from build123d import *

# Parameters (mm, degrees)
CROQUIS1_W              = 56
CROQUIS1_H              = 56
CROQUIS1_R              = 4
CROQUIS1_R_2            = 1.6
SALIENTE_EXTRUIR1_DEPTH = 5
CROQUIS2_W              = 56
CROQUIS2_H              = 3
SALIENTE_EXTRUIR2_DEPTH = 20
CROQUIS3_R              = 4.2
CORTAR_EXTRUIR1_DEPTH   = 68.416615163
CROQUIS4_R              = 2.75
CORTAR_EXTRUIR2_DEPTH   = 3
CROQUIS7_W              = 8
CROQUIS7_H              = 10
SALIENTE_EXTRUIR3_DEPTH = 5
CROQUIS5_R              = 5
CORTAR_EXTRUIR3_DEPTH   = 47.829477896
CHAFL_N1_SIZE           = 2
CHAFL_N2_SIZE           = 1.5


with BuildPart() as part:
    # Croquis1 → Saliente-Extruir1 (new body)
    with BuildSketch(Plane.XY):
        Rectangle(CROQUIS1_W, CROQUIS1_H)
        Circle(CROQUIS1_R, mode=Mode.SUBTRACT)
        with Locations((0, 11)):
            Circle(CROQUIS1_R_2, mode=Mode.SUBTRACT)
        with Locations((11, 0)):
            Circle(CROQUIS1_R_2, mode=Mode.SUBTRACT)
        with Locations((0, -11)):
            Circle(CROQUIS1_R_2, mode=Mode.SUBTRACT)
        with Locations((-11, 0)):
            Circle(CROQUIS1_R_2, mode=Mode.SUBTRACT)
    extrude(amount=SALIENTE_EXTRUIR1_DEPTH)

    # Croquis2 → Saliente-Extruir2 (add)
    with BuildSketch(Plane.XY.offset(5)):
        with Locations((0, 26.5)):
            Rectangle(CROQUIS2_W, CROQUIS2_H)
        with Locations((0, -26.5)):
            Rectangle(CROQUIS2_W, CROQUIS2_H)
    extrude(amount=SALIENTE_EXTRUIR2_DEPTH)

    # Croquis3 → Cortar-Extruir1 (cut, through all)
    with BuildSketch(Plane(origin=(0, 28, 0), x_dir=(1, 0, 0), z_dir=(0, 1, 0))):
        with Locations(Location((0, -15, 0), (0, 0, 270))):
            Circle(CROQUIS3_R)
    extrude(amount=-CORTAR_EXTRUIR1_DEPTH, mode=Mode.SUBTRACT)

    # Croquis4 → Cortar-Extruir2 (cut)
    with BuildSketch(Plane.XY.offset(5)):
        with Locations((-11, 0)):
            Circle(CROQUIS4_R)
        with Locations((0, 11)):
            Circle(CROQUIS4_R)
        with Locations((11, 0)):
            Circle(CROQUIS4_R)
        with Locations((0, -11)):
            Circle(CROQUIS4_R)
    extrude(amount=-CORTAR_EXTRUIR2_DEPTH, mode=Mode.SUBTRACT)

    # Croquis7 → Saliente-Extruir3 (add)
    with BuildSketch(Plane.XY.offset(5)):
        with Locations((-24, 0)):
            Rectangle(CROQUIS7_W, CROQUIS7_H)
    saliente_extruir3 = extrude(amount=SALIENTE_EXTRUIR3_DEPTH)

    # Simetría2: Saliente-Extruir3 across plane
    add(saliente_extruir3.mirror(Plane(origin=(0, 0, 0), x_dir=(0, 0, 1), z_dir=(1, 0, 0))))

    # Croquis5 → Cortar-Extruir3 (cut, through all)
    with BuildSketch(Plane(origin=(0, 0, 0), x_dir=(-1, 0, 0), z_dir=(0, 0, -1))):
        with Locations((20, 0)):
            Circle(CROQUIS5_R)
    cortar_extruir3 = extrude(amount=-CORTAR_EXTRUIR3_DEPTH, mode=Mode.SUBTRACT)

    # Simetría1: Cortar-Extruir3 across plane
    add(cortar_extruir3.mirror(Plane(origin=(0, 0, 0), x_dir=(0, 0, 1), z_dir=(1, 0, 0))), mode=Mode.SUBTRACT)

    # Chaflán1
    chafl_n1_edges = [part.edges().sort_by_distance(p)[0] for p in [
        (-28, 28, 12.5),
        (28, 28, 12.5),
        (28, -28, 12.5),
        (-28, -28, 12.5),
    ]]
    chamfer(chafl_n1_edges, length=CHAFL_N1_SIZE)

    # Chaflán2
    chafl_n2_edges = [part.edges().sort_by_distance(p)[0] for p in [
        (28, 0, 0),
        (-28, 0, 0),
        (0, 28, 0),
        (0, -28, 0),
        (-27, 27, 0),
        (-27, -27, 0),
        (27, 27, 0),
        (27, -27, 0),
    ]]
    chamfer(chafl_n2_edges, length=CHAFL_N2_SIZE)


solid = part.part
Here's how the part is built. I have some questions about the finished solid (model axes, mm). A direction names the side the tool comes from. Round coordinates to 2 decimals unless told otherwise and drop trailing zeros. Write each loop counter-clockwise with the first axis right and the second up, starting at its lowest first coordinate (ties: lowest second). Pieces come first, ordered by that corner, then holes.
1. Suppose I cut it at D-D (y = 11). List the corners of the cut face in (x, z) for me.
2. For faces 1 (the flat face through (26, 0, 10)), 2 (the flat face through (-26.476, 26.448, 0.74)), 3 (the cylindrical face through (-2.027, -9.141, 3.521)), which set-ups out of +Z, -Z, +X, -X, +Y, -Y let a thin tool reach every point of the face, with its end or its side?
3. I need wall thicknesses on L1, parallel to Y at x = 0, z = 3.05; L2, parallel to Y at x = 6, z = 15. Which ranges of each line are inside material? Lowest first, please.
4. Will these pins go through, and if not, where does the flat tip stop? pin 1 Ø9 at (x, y) = (-26, 0) entering from +Z; pin 2 Ø3 at (x, y) = (-21, 21.5) entering from +Z.
5. Suppose I cut it at B-B (x = 11). List the corners of the cut face in (y, z) for me.
6. Suppose I cut it at C-C (y = 0). State how many separate pieces and enclosed holes the cut face has, and give its area (3 significant figures).
7. If we mould it in two halves opening along Y, with no side actions, what happens to faces 4 (the flat face through (-27, 27, 13)), 5 (the cylindrical face through (-24.77, 1.5, 3.82)), 6 (the flat face through (0, -28, 10))? For each: released by +Y, released by -Y, zero draft, split by the parting line, or undercut.
8. Suppose I cut it at A-A (z = 23). List the corners of the cut face in (x, y) for me, and give its area (3 significant figures).
Answer sheet:
1. outline: (-28, 1.5) - (-26.5, 0) - (-1.6, 0) - (-1.6, 2) - (-2.75, 2) - (-2.75, 5) - (-28, 5) - close; (1.6, 0) - (26.5, 0) - (28, 1.5) - (28, 5) - (2.75, 5) - (2.75, 2) - (1.6, 2) - close
2. face 1: +Z, +X, -X
2. face 2: -Z, -X, +Y
2. face 3: +Z
3. L1: y = -28 to -13.75, -8.25 to -4, 4 to 8.25, 13.75 to 28
3. L2: y = -28 to -25, 25 to 28
4. pin 1: stops at z = 10
4. pin 2: stops at z = 5
5. outline: (-28, 1.5) - (-26.5, 0) - (-1.6, 0) - (-1.6, 2) - (-2.75, 2) - (-2.75, 5) - (-25, 5) - (-25, 25) - (-28, 25) - close; (1.6, 0) - (26.5, 0) - (28, 1.5) - (28, 25) - (25, 25) - (25, 5) - (2.75, 5) - (2.75, 2) - (1.6, 2) - close
6. separate pieces: 6
6. enclosed holes: 0
6. area: 122 mm2
7. face 4: released by +Y
7. face 5: undercut
7. face 6: released by -Y
8. outline: (-28, -26) - (-26, -28) - (26, -28) - (28, -26) - (28, -25) - (-28, -25) - close; (-28, 25) - (28, 25) - (28, 26) - (26, 28) - (-26, 28) - (-28, 26) - close
8. area: 328 mm2
